```python
from build123d import *

# Parameters (mm, degrees)
SALIENTE_EXTRUIR1_DEPTH = 8
REDONDEO1_R             = 1
CROQUIS2_R              = 1.125
CORTAR_EXTRUIR1_DEPTH   = 18
CROQUIS3_R              = 1.125
CORTAR_EXTRUIR2_DEPTH   = 18
REDONDEO2_R             = 1


with BuildPart() as part:
    # Croquis1 → Saliente-Extruir1 (new body)
    with BuildSketch(Plane(origin=(0, 0, 0), x_dir=(0, 0, -1), z_dir=(1, 0, 0))):
        Polygon((0, 0), (0, 12), (12, 12), (12, 9), (3, 9), (3, 0), align=None)
    extrude(amount=SALIENTE_EXTRUIR1_DEPTH)

    # Redondeo1
    redondeo1_edges = [part.edges().sort_by_distance(p)[0] for p in [
        (8, 10.5, -12),
        (8, 0, -1.5),
        (0, 10.5, -12),
        (0, 0, -1.5),
    ]]
    fillet(redondeo1_edges, radius=REDONDEO1_R)

    # Croquis2 → Cortar-Extruir1 (cut, through all)
    with BuildSketch(Plane.XZ.offset(-9)):
        with Locations(Location((4, -7.519001503, 0), (0, 0, 270))):
            Circle(CROQUIS2_R)
    extrude(amount=-CORTAR_EXTRUIR1_DEPTH, mode=Mode.SUBTRACT)

    # Croquis3 → Cortar-Extruir2 (cut, through all)
    with BuildSketch(Plane(origin=(0, 0, -3), x_dir=(-1, 0, 0), z_dir=(0, 0, -1))):
        with Locations(Location((-4, 4.480998497, 0), (0, 0, 90))):
            Circle(CROQUIS3_R)
    extrude(amount=-CORTAR_EXTRUIR2_DEPTH, mode=Mode.SUBTRACT)

    # Redondeo2
    redondeo2_edges = [part.edges().sort_by_distance(p)[0] for p in [
        (4, 12, 0),
    ]]
    fillet(redondeo2_edges, radius=REDONDEO2_R)


solid = part.part
```
Geometry check sheet. Reference: the model listing, model coordinates, mm. A direction names the side the tool comes from. Coordinates: 2 decimals unless noted, no trailing zeros. Order: outer loops, then holes, each group sorted by start corner. A loop starts at its lowest first (then second) coordinate and runs counter-clockwise, first axis right, second up.
Item 1: Section check B-B (z = -7). Enter the section's corners in (x, y), plus the area to 3 significant figures.
Item 2: Mould release check, pull along X, two halves, no side actions. Record for faces 3 (the flat face through (0, 10, -4)), 4 (the flat face through (4, 0, -2)), 5 (the flat face through (8, 10, -4)), 6 (the cylindrical face through (5, 10, -7)): released by +X, released by -X, zero draft, split by the parting line, or undercut.
Item 3: Section check D-D (x = 1.75). Enter the section's corners in (y, z), plus the area to 3 significant figures.
Item 4: Depth check by flat-ended pin: pin 1 (2 mm diameter, centred on x = 4.5, y = 7.5, fed in from -Z); pin 2 (3 mm diameter, centred on x = 4.5, z = -9, fed in from -Y). Enter the tip coordinate at first touch or a pass-through.
Item 5: Tool access check on faces 1 (the flat face through (3.1, 9, -6.6)), 2 (the flat face through (4, 11, -12)). Record the directions out of +Z, -Z, +X, -X, +Y, -Y that give a thin tool (end or side, any length) a straight path to the whole face; none if there is none.
Item 6: Section check C-C (y = 5.25). Enter the section's corners in (x, z), plus the area to 3 significant figures.
Item 7: Scan lines: line 1 along Y through (x, z) = (2.5, -6.75); line 2 along Z through (x, y) = (7.25, 6.25); line 3 along X through (y, z) = (10, -8). Record each from-to range of solid material in increasing order.
Item 8: Section check A-A (x = 4). Enter the section's corners in (y, z).
Check sheet entries:
1. outline: (0, 9) - (3, 9) - (3, 12) - (0, 12) - close; (5, 9) - (8, 9) - (8, 12) - (5, 12) - close
1. area: 18.0 mm2
2. face 3: released by -X
2. face 4: zero draft
2. face 5: released by +X
2. face 6: undercut
3. outline: (0, -3) - (9, -3) - (9, -12) - (12, -12) - (12, -1) arc R1 ccw to (11, 0) - (0, 0) - close
3. area: 62.8 mm2
4. pin 1: stops at z = -3
4. pin 2: stops at y = 9
5. face 1: -Z, +X, -X, -Y
5. face 2: -Z, +X, -X, +Y, -Y
6. outline: (0, -3) - (3.18, -3) - (3.18, 0) - (0, 0) - close; (4.82, -3) - (8, -3) - (8, 0) - (4.82, 0) - close
6. area: 19.1 mm2
7. line 1: y = 9 to 12
7. line 2: z = -3 to 0
7. line 3: x = 0 to 2.98, 5.02 to 8
8. outline: (0, -3) - (3.36, -3) - (3.36, 0) - (0, 0) - close; (5.61, -3) - (9, -3) - (9, -6.39) - (12, -6.39) - (12, -1) arc R1 ccw to (11, 0) - (5.61, 0) - close; (9, -12) - (12, -12) - (12, -8.64) - (9, -8.64) - close
